from build123d import *

# Parameters (mm, degrees)
F0_W      = 76.2
F0_H      = 25.4
F1_DEPTH  = 12.7
F3_DEPTH  = 25.4
F4_W      = 25.4
F4_H      = 25.4
F5_DEPTH  = 31.75
F7_DEPTH  = 25.4
F8_R      = 6.35
F9_DEPTH  = 12.7
F10_R     = 6.35
F11_DEPTH = 25.4


with BuildPart() as f1:
    # F0 (on Top) → F1 (new body)
    with BuildSketch(Plane.XY):
        with Locations((38.1, 12.7)):
            Rectangle(F0_W, F0_H)
    extrude(amount=F1_DEPTH)

    # F2 (on face) → F3 (cut)
    with BuildSketch(Plane.XY.offset(12.7)):
        with BuildLine():
            ThreePointArc((6.35, 0), (0.081424, 12.7), (6.35, 25.4))
            Line((6.35, 25.4), (0, 25.4))
            Line((0, 25.4), (0, 0))
            Line((0, 0), (6.35, 0))
        make_face()
        with BuildLine():
            Line((76.2, 25.4), (69.85, 25.4))
            ThreePointArc((69.85, 25.4), (76.079165, 12.7), (69.85, 0))
            Line((69.85, 0), (76.2, 0))
            Line((76.2, 0), (76.2, 25.4))
        make_face()
    extrude(amount=-F3_DEPTH, mode=Mode.SUBTRACT)

    # F4 (on face) → F5 (join)
    with BuildSketch(Plane.XY.offset(12.7)):
        with Locations((38.1, 12.7)):
            Rectangle(F4_W, F4_H)
    extrude(amount=F5_DEPTH)

    # F6 (on face) → F7 (cut)
    with BuildSketch(Plane.YZ.offset(50.8)):
        with BuildLine():
            Line((0, 44.45), (0, 38.1))
            ThreePointArc((0, 38.1), (12.7, 44.313005), (25.4, 38.1))
            Line((25.4, 38.1), (25.4, 44.45))
            Line((25.4, 44.45), (0, 44.45))
        make_face()
    extrude(amount=-F7_DEPTH, mode=Mode.SUBTRACT)

    # F8 (on face) → F9 (cut)
    with BuildSketch(Plane.XY.offset(12.7)):
        with Locations((12.781424, 12.7)):
            Circle(F8_R)
        with Locations((63.5, 12.7)):
            Circle(F8_R)
    extrude(amount=-F9_DEPTH, mode=Mode.SUBTRACT)

    # F10 (on face) → F11 (cut)
    with BuildSketch(Plane.YZ.offset(50.8)):
        with Locations((12.7, 31.613005)):
            Circle(F10_R)
    extrude(amount=-F11_DEPTH, mode=Mode.SUBTRACT)


solid = f1.part
Work out the finished part from the listing and answer in its coordinate system (mm). A direction names the side the tool comes from. Give positions to 0.01 mm unless a question says otherwise; leave off trailing zeros. Write each loop counter-clockwise with the first axis right and the second up, starting at its lowest first coordinate (ties: lowest second). Pieces come first, ordered by that corner, then holes.
Q1. The part is cut by section B-B on y = 12.7. Give the vertices of the cut face in (x, z), and give its area (3 significant figures).
Answer:
outline: (0.08, 0) - (6.43, 0) - (6.43, 12.7) - (0.08, 12.7) - close; (19.13, 0) - (57.15, 0) - (57.15, 12.7) - (50.8, 12.7) - (50.8, 25.26) - (25.4, 25.26) - (25.4, 12.7) - (19.13, 12.7) - close; (25.4, 37.96) - (50.8, 37.96) - (50.8, 44.31) - (25.4, 44.31) - close; (69.85, 0) - (76.08, 0) - (76.08, 12.7) - (69.85, 12.7) - close
area: 1,120 mm2
Q2. For a pull along Y with two mould halves and no side action, classify faces 1 (the face through (16.2, 18.05, 6.44)), 2 (the face through (38, 25.4, 15)), 3 (the face through (50.8, 13, 25)), 4 (the face through (0.083, 12.495, 6.439)) as released by +Y, released by -Y, zero draft, split by the parting line, or undercut.
Answer:
face 1: undercut
face 2: released by +Y
face 3: zero draft
face 4: split by the parting line
Q3. The part is cut by section D-D on y = 5.5. Give the vertices of the cut face in (x, z).
Answer:
outline: (1.79, 0) - (74.37, 0) - (74.37, 12.7) - (50.8, 12.7) - (50.8, 42.61) - (25.4, 42.61) - (25.4, 12.7) - (1.79, 12.7) - close
Q4. Given pin 1 (1.5 mm diameter, centred on x = 47, y = 14.5, fed in from +Z); pin 2 (14.5 mm diameter, centred on y = 12.7, z = 31.61, fed in from +X); pin 3 (6 mm diameter, centred on x = 13, y = 2.5, fed in from -Z); pin 4 (6 mm diameter, centred on x = 8, y = 4.5, fed in from +Z), each flat-ended and moving along its own axis, determine where each tip first touches the part or whether it passes through.
Answer:
pin 1: stops at z = 44.28
pin 2: stops at x = 50.8
pin 3: stops at z = 0
pin 4: stops at z = 12.7
Q5. Straight lines are drawn through the part: L1, parallel to Z at x = 38, y = 12.7; L2, parallel to X at y = 18.75, z = 41; L3, parallel to Y at x = 63.5, z = 6.25. For each, find the intervals that lie inside material, in ascending order.
Answer:
L1: z = 0 to 25.26, 37.96 to 44.31
L2: x = 25.4 to 50.8
L3: y = 0 to 6.35, 19.05 to 25.4
Q6. The part is cut by section C-C on z = 37. Give the vertices of the cut face in (x, y).
Answer:
outline: (25.4, 0) - (50.8, 0) - (50.8, 9.34) - (25.4, 9.34) - close; (25.4, 16.06) - (50.8, 16.06) - (50.8, 25.4) - (25.4, 25.4) - close
Q7. A tool of negligible diameter and unlimited length cuts with its end or side. For faces 5 (the face through (57.6, 15.7, 12.7)), 6 (the face through (38.28, 12.5, 44.31)), 7 (the face through (25.4, 13, 25)), from which of +Z, -Z, +X, -X, +Y, -Y can it reach the whole face along a straight path? Write none if from no direction.
Answer:
face 5: +Z, +X, +Y, -Y
face 6: +Z, +X, -X
face 7: +Z, -X, +Y, -Y
Q8. The part is cut by section A-A on x = 63.5. Give the vertices of the cut face in (y, z), and give its area (3 significant figures).
Answer:
outline: (0, 0) - (6.35, 0) - (6.35, 12.7) - (0, 12.7) - close; (19.05, 0) - (25.4, 0) - (25.4, 12.7) - (19.05, 12.7) - close
area: 161 mm2
